```python
from build123d import *

# Parameters (mm, degrees)
SKETCH_1_W          = 9
SKETCH_1_H          = 12
EXTRUDE_1_DEPTH     = 28
SKETCH_2_OUTSIDE_W  = 20.352
SKETCH_2_OUTSIDE_H  = 36.352
CUT_EXTRUDE_1_DEPTH = 31.01666204
SKETCH_3_R          = 3
CUT_EXTRUDE_2_DEPTH = 10
SKETCH_4_R          = 3
CUT_EXTRUDE_3_DEPTH = 30.978055751


with BuildPart() as part:
    # 草图1 → 凸台-拉伸1 (new body)
    with BuildSketch(Plane(origin=(0, 0, 0), x_dir=(1, 0, 0), z_dir=(0, 1, 0))):
        Rectangle(SKETCH_1_W, SKETCH_1_H)
    extrude(amount=EXTRUDE_1_DEPTH)

    # 草图2 outside → 切除-拉伸1 (cut, through all)
    with BuildSketch(Plane(origin=(4.5, 0, 0), x_dir=(0, 0, -1), z_dir=(1, 0, 0))):
        with Locations((0, 14)):
            Rectangle(SKETCH_2_OUTSIDE_W, SKETCH_2_OUTSIDE_H)
        with BuildLine():
            Line((-6, -3.744960893), (-6, 21.958609168))
            ThreePointArc((-6, 21.958609168), (0, 27.958609168), (6, 21.958609168))
            Line((6, 21.958609168), (6, -3.744960893))
            ThreePointArc((6, -3.744960893), (0, -9.744960893), (-6, -3.744960893))
        make_face(mode=Mode.SUBTRACT)
    extrude(amount=-CUT_EXTRUDE_1_DEPTH, mode=Mode.SUBTRACT)

    # 草图3 → 切除-拉伸2 (cut)
    with BuildSketch(Plane.XZ):
        with Locations(Location((0, 0, 0), (0, 0, 270))):
            Circle(SKETCH_3_R)
    extrude(amount=-CUT_EXTRUDE_2_DEPTH, mode=Mode.SUBTRACT)

    # 草图4 → 切除-拉伸3 (cut, through all)
    with BuildSketch(Plane(origin=(4.5, 0, 0), x_dir=(0, 0, -1), z_dir=(1, 0, 0))):
        with Locations((0, 21.958609168)):
            Circle(SKETCH_4_R)
    extrude(amount=-CUT_EXTRUDE_3_DEPTH, mode=Mode.SUBTRACT)


solid = part.part
```
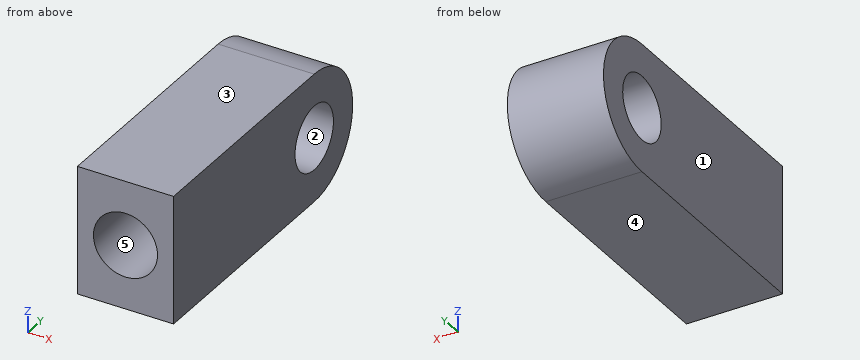
CAD build for the part. Positions are in the model's coordinates, mm. Face numbers are marked on the shaded views. A direction names the side the tool comes from. Round coordinates to 2 decimals unless told otherwise and drop trailing zeros. Order: outer loops, then holes, each group sorted by start corner. A loop starts at its lowest first (then second) coordinate and runs counter-clockwise, first axis right, second up. Notation, with made-up numbers: (78.5, 72.5) - (126.5, 72.5) arc R28 ccw to (126.5, 98.5) - close; hole circle Ø9 at (85, 61). An arc over 180 degrees is marked (long way). Answer in a Markdown table with one row per item. Add a question column.
(1) Mould opens along Z. For the marked faces 1, 2 and 3 say: +Z half, -Z half, draft (parallel to the pull), parting line (faces both ways), or undercut.
(2) Band-saw the part on A-A on y = 7. List the corners of the cut face in (x, z), and give its area (3 significant figures).
(3) Probe L1, parallel to X at y = 9, z = 0; L2, parallel to X at y = 7.5, z = -1.5; L3, parallel to Y at x = -3, z = -2.5. List the from-to ranges inside material, lowest first. Write a range as [from, to].
(4) Band-saw the part on C-C on z = 0. List the corners of the cut face in (x, y).
(5) Drop flat-ended pins along their axis: pin 1 Ø5 at (x, z) = (3, 4.5) entering from -Y; pin 2 Ø2 at (x, z) = (-3, -1.5) entering from +Y. Give the stop position or say it passes through.
(6) Band-saw the part on D-D on y = 22.5. List the corners of the cut face in (x, z).
(7) Band-saw the part on B-B on x = 0. List the corners of the cut face in (y, z), and give its area (3 significant figures).
(8) 3-axis set-ups, long thin cutter, end or side, ignore diameter. For the marked faces 4 and 5: which of +Z, -Z, +X, -X, +Y, -Y reach the whole face in a straight line?
Data:
| question | item | result |
|---|---|---|
| 1 | face 1 | draft |
| 1 | face 2 | undercut |
| 1 | face 3 | +Z half |
| 2 | outline | (-4.5, -6) - (4.5, -6) - (4.5, 6) - (-4.5, 6) - close; hole circle Ø6 at (0, 0) |
| 2 | area | 79.7 mm^2 |
| 3 | L1 | x = [-4.5, -3], [3, 4.5] |
| 3 | L2 | x = [-4.5, -2.6], [2.6, 4.5] |
| 3 | L3 | y = [0, 20.3], [23.62, 27.41] |
| 4 | outline | (-4.5, 0) - (-3, 0) - (-3, 10) - (3, 10) - (3, 0) - (4.5, 0) - (4.5, 18.96) - (-4.5, 18.96) - close; (-4.5, 24.96) - (4.5, 24.96) - (4.5, 27.96) - (-4.5, 27.96) - close |
| 5 | pin 1 | stops at y = 0 |
| 5 | pin 2 | stops at y = 27.94 |
| 6 | outline | (-4.5, -5.98) - (4.5, -5.98) - (4.5, -2.95) - (-4.5, -2.95) - close; (-4.5, 2.95) - (4.5, 2.95) - (4.5, 5.98) - (-4.5, 5.98) - close |
| 7 | outline | (0, -6) - (21.96, -6) arc R6 ccw to (21.96, 6) - (0, 6) - (0, 3) - (10, 3) - (10, -3) - (0, -3) - close; hole circle Ø6 at (21.96, 0) |
| 7 | area | 232 mm^2 |
| 8 | face 4 | -Z, +X, -X, +Y, -Y |
| 8 | face 5 | -Y |
